For this review, take the finished solid that the model builds, in its own axes (mm). A direction names the side the tool comes from. Give positions to 0.01 mm unless a question says otherwise; leave off trailing zeros. Loops run counter-clockwise (first coordinate to the right, second up) from the corner with the lowest first, then second, coordinate; pieces in that order, holes last. Notation, with made-up numbers: M -7,71 L 2,71 A23 ccw 2,92 Z; hole C 76.5,25.25 d5. An arc over 180 degrees is marked long. Use CSV: the item, a comma, the result in double quotes. Start each with the question number.
1. Tool access review of faces 1 (the face through (19, 5, -56.45)), 2 (the face through (19, 1.67, -62)), 3 (the face through (9.35, 5, -61)): name each direction out of +Z, -Z, +X, -X, +Y, -Y from which nothing blocks a thin tool from reaching the whole face with its end or side.
2. Take a section at A-A, the plane y = 3. Write out the cut boundary in (x, z).
3. Take a section at D-D, the plane y = 7. Write out the cut boundary in (x, z).
4. To check wall thickness, follow line 1 (Z direction, x = 37, y = 1.5); line 2 (X direction, y = 2.75, z = -60.5); line 3 (Y direction, x = 12.5, z = -45). State the ranges of each line that lie inside material, in increasing order. Write a range as [from, to].
5. Insertion check: P1, Ø1.5, axis at y = 6, z = -55.5, coming from the +X side; P2, Ø3, axis at y = 5.5, z = -58.5, coming from the +X side; P3, Ø0.6, axis at y = 3, z = -52.5, coming from the +X side; P4, Ø1.1, axis at y = 3, z = -52.5, coming from the -X side. Each pin has a flat end and moves straight along its axis. Give the tip position at first contact, or say it passes through.
6. Take a section at C-C, the plane x = 19. Write out the cut boundary in (y, z).
7. Take a section at B-B, the plane z = -48. Write out the cut boundary in (x, y).
from build123d import *

# Parameters (mm, degrees)
SKETCH1_W           = 39.63
SKETCH1_H           = 59.15
BOSS_EXTRUDE1_DEPTH = 1.67
BOSS_EXTRUDE2_START = 1.67
SKETCH2_W           = 20.25
SKETCH2_H           = 8.65
BOSS_EXTRUDE2_DEPTH = 6
SKETCH3_W           = 4.67
SKETCH3_H           = 11.2
BOSS_EXTRUDE3_DEPTH = 3.8


with BuildPart() as part:
    # Sketch1 → Boss-Extrude1 (new body)
    with BuildSketch(Plane(origin=(0, 0, 0), x_dir=(1, 0, 0), z_dir=(0, 1, 0))):
        with Locations((19.815, 29.575)):
            Rectangle(SKETCH1_W, SKETCH1_H)
    extrude(amount=BOSS_EXTRUDE1_DEPTH)

    # Sketch2 → Boss-Extrude2 (add)
    with BuildSketch(Plane(origin=(0, 0, 0), x_dir=(1, 0, 0), z_dir=(0, 1, 0)).offset(BOSS_EXTRUDE2_START)):
        with Locations((19.475, 60.775)):
            Rectangle(SKETCH2_W, SKETCH2_H)
    extrude(amount=BOSS_EXTRUDE2_DEPTH)

    # Sketch3 → Boss-Extrude3 (add)
    with BuildSketch(Plane(origin=(0, 0, 0), x_dir=(1, 0, 0), z_dir=(0, 1, 0))):
        with Locations((36.835, 52.35)):
            Rectangle(SKETCH3_W, SKETCH3_H)
    extrude(amount=BOSS_EXTRUDE3_DEPTH)


solid = part.part
Result set:
1,face 1,"+Z, -X, +Y"
1,face 2,"-Z, +X, -X, -Y"
1,face 3,"+Z, -Z, -X, +Y"
2,outline,"M 9.35,-65.1 L 29.6,-65.1 L 29.6,-56.45 L 9.35,-56.45 Z; M 34.5,-57.95 L 39.17,-57.95 L 39.17,-46.75 L 34.5,-46.75 Z"
3,outline,"M 9.35,-65.1 L 29.6,-65.1 L 29.6,-56.45 L 9.35,-56.45 Z"
4,line 1,"[-59.15, 0]"
4,line 2,"[9.35, 29.6]"
4,line 3,"[0, 1.67]"
5,P1,"through"
5,P2,"x = 29.6"
5,P3,"x = 39.17"
5,P4,"x = 34.5"
6,outline,"M 0,-59.15 L 1.67,-59.15 L 1.67,-65.1 L 7.67,-65.1 L 7.67,-56.45 L 1.67,-56.45 L 1.67,0 L 0,0 Z"
7,outline,"M 0,0 L 39.63,0 L 39.63,1.67 L 39.17,1.67 L 39.17,3.8 L 34.5,3.8 L 34.5,1.67 L 0,1.67 Z"
